```python
from build123d import *

# Parameters (mm, degrees)
SKETCH_1_W   = 15
SKETCH_1_H   = 3
SKETCH_1_W_2 = 10
SKETCH_1_H_2 = 20


with BuildPart() as part:
    # 草圖1 → 旋轉1 (revolve)
    with BuildSketch(Plane.XY, mode=Mode.PRIVATE) as revolve_1_sk:
        with Locations((-7.5, 1.5)):
            Rectangle(SKETCH_1_W, SKETCH_1_H)
        with Locations((-5, 13)):
            Rectangle(SKETCH_1_W_2, SKETCH_1_H_2)
        Polygon((-10, 23), (0, 23), (0, 26), (-15, 26), (-15, 23), align=None)
    revolve(revolve_1_sk.sketch.rotate(Axis((0, 0, 0), (0, 1, 0)), 270), axis=Axis((0, 0, 0), (0, 1, 0)))


solid = part.part
```
Here's how the part is built. I have some questions about the finished solid (model axes, mm). A direction names the side the tool comes from. Coordinates: 2 decimals unless noted, no trailing zeros. Order: outer loops, then holes, each group sorted by start corner. A loop starts at its lowest first (then second) coordinate and runs counter-clockwise, first axis right, second up. Notation, with made-up numbers: (29.25, 31) - (80.25, 31) arc R15 cw to (80.25, 49) - close; hole circle Ø10 at (32, 19). An arc over 180 degrees is marked (long way). One line per question, with ' | ' between items. Start each with the question number.
1. I'm going to push flat-ended pins straight in: pin 1 Ø4 at (y, z) = (11.5, -11) entering from +X; pin 2 Ø2 at (x, y) = (-10, 10) entering from +Z; pin 3 Ø5 at (x, y) = (2.5, 9.5) entering from +Z; pin 4 Ø9 at (x, z) = (4, 4) entering from -Y. Where does each tip first touch, or does it pass through?
2. If we section it at A-A (z = 10.75): Write out the boundary of the cut face in (x, y).
3. Which directions (+Z, -Z, +X, -X, +Y, -Y) give clear straight access to the entire face, cutting with the end or side of a thin tool? Please do faces 1 (the flat face through (0, 0, 0)), 2 (the flat face through (3, 23, -10)).
4. If we mould it in two halves opening along Y, with no side actions, what happens to faces 3 (the cylindrical face through (9.76, 13.14, 2.17)), 4 (the cylindrical face through (-0.66, 24.479, 14.985)), 5 (the flat face through (0, 26, 0))? For each: released by +Y, released by -Y, zero draft, split by the parting line, or undercut.
5. If we section it at B-B (x = 0): Write out the boundary of the cut face in (y, z).
6. If we section it at C-C (z = 0): Write out the boundary of the cut face in (x, y).
7. Please list where these lines run through material, in increasing order: line 1 along Y through (x, z) = (8.25, -8.5); line 2 along Z through (x, y) = (1, 10.5); line 3 along Z through (x, y) = (5.75, 18.5). Write a range as [from, to].
8. If we section it at D-D (y = 2.25): Write out the boundary of the cut face in (x, z), and give its area (3 significant figures).
Model answer:
1) pin 1: stops at x = 4.36 | pin 2: stops at z = 4.36 | pin 3: stops at z = 10 | pin 4: stops at y = 0
2) outline: (-10.46, 0) - (10.46, 0) - (10.46, 3) - (-10.46, 3) - close; (-10.46, 23) - (10.46, 23) - (10.46, 26) - (-10.46, 26) - close
3) face 1: +Z, -Z, +X, -X, -Y | face 2: none
4) face 3: undercut | face 4: zero draft | face 5: released by +Y
5) outline: (0, -15) - (3, -15) - (3, -10) - (23, -10) - (23, -15) - (26, -15) - (26, 15) - (23, 15) - (23, 10) - (3, 10) - (3, 15) - (0, 15) - close
6) outline: (-15, 0) - (15, 0) - (15, 3) - (10, 3) - (10, 23) - (15, 23) - (15, 26) - (-15, 26) - (-15, 23) - (-10, 23) - (-10, 3) - (-15, 3) - close
7) line 1: y = [0, 3], [23, 26] | line 2: z = [-9.95, 9.95] | line 3: z = [-8.18, 8.18]
8) outline: circle Ø30 at (0, 0) | area: 707 mm²
